Source: CAD feature listing. Evaluate the final solid. Frame: model axes, mm. Give positions to 0.01 mm unless a question says otherwise; leave off trailing zeros. Loops run counter-clockwise (first coordinate to the right, second up) from the corner with the lowest first, then second, coordinate; pieces in that order, holes last. Notation, with made-up numbers: (52.25, 53) - (64.25, 53) arc R32 cw to (64.25, 79) - close; hole circle Ø4 at (1, -21.75). An arc over 180 degrees is marked (long way). Put each result on its own line as item: value.
```python
from build123d import *

# Parameters (mm, degrees)
F0_R     = 7.5
F0_R_2   = 5
F1_DEPTH = 6


with BuildPart() as f1:
    # F0 (on Front) → F1 (new body)
    with BuildSketch(Plane.XZ):
        with BuildLine():
            ThreePointArc((-230, 50), (-244.142136, 44.142136), (-250, 30))
            Line((-250, 30), (-250, -30))
            ThreePointArc((-250, -30), (-244.142136, -44.142136), (-230, -50))
            Line((-230, -50), (230, -50))
            ThreePointArc((230, -50), (244.142136, -44.142136), (250, -30))
            Line((250, -30), (250, 30))
            ThreePointArc((250, 30), (244.142136, 44.142136), (230, 50))
            Line((230, 50), (-230, 50))
        make_face()
        with Locations((-225, 0)):
            Circle(F0_R, mode=Mode.SUBTRACT)
        Circle(F0_R_2, mode=Mode.SUBTRACT)
        with Locations((225, 0)):
            Circle(F0_R, mode=Mode.SUBTRACT)
    extrude(amount=F1_DEPTH)


solid = f1.part
```
1) Section query C-C, the plane y = -3.2. Output: boundary loops of the cut face in (x, z), plus the area to 3 significant figures.
Check result:
outline: (-250, -30) arc R20 ccw to (-230, -50) - (230, -50) arc R20 ccw to (250, -30) - (250, 30) arc R20 ccw to (230, 50) - (-230, 50) arc R20 ccw to (-250, 30) - close; hole circle Ø15 at (-225, 0); hole circle Ø10 at (0, 0); hole circle Ø15 at (225, 0)
area: 49,200 mm²
2) Section query D-D, the plane x = -225. Output: boundary loops of the cut face in (y, z), plus the area to 3 significant figures.
Check result:
outline: (-6, -50) - (0, -50) - (0, -7.5) - (-6, -7.5) - close; (-6, 7.5) - (0, 7.5) - (0, 50) - (-6, 50) - close
area: 510 mm²
3) Pin query (flat end, axial travel): P1, Ø12, axis at x = -193, z = -7, coming from the +Y side; P2, Ø1.5, axis at y = -3, z = 36.5, coming from the +X side. Return the tip coordinate at first contact, or that it passes through.
Check result:
P1: y = 0
P2: x = 249.16
4) Section query A-A, the plane x = 0. Output: boundary loops of the cut face in (y, z).
Check result:
outline: (-6, -50) - (0, -50) - (0, -5) - (-6, -5) - close; (-6, 5) - (0, 5) - (0, 50) - (-6, 50) - close
5) Material intervals for line 1 along Z through (x, y) = (-225, -3.2); line 2 along Z through (x, y) = (0, -2.4); line 3 along X through (y, z) = (-5.6, 31), sorted ascending. Write a range as [from, to].
Check result:
line 1: [-50, -7.5], [7.5, 50]
line 2: [-50, -5], [5, 50]
line 3: [-249.97, 249.97]
6) Mould query, pull axis Z, two halves, no side actions, for faces 1 (the cylindrical face through (217.507, -2.958, 0.33)), 2 (the cylindrical face through (-244.297, -2.958, -43.986)), 3 (the cylindrical face through (-1.08, -2.96, -4.88)), 4 (the cylindrical face through (-243.986, -2.958, 44.297)). Classes: pulls with the +Z half, pulls with the -Z half, needs draft (parallel to the pull), parting line crosses it, or undercut.
Check result:
face 1: undercut
face 2: pulls with the -Z half
face 3: undercut
face 4: pulls with the +Z half
7) Section query B-B, the plane z = 0. Output: boundary loops of the cut face in (x, y), plus the area to 3 significant figures.
Check result:
outline: (-250, -6) - (-232.5, -6) - (-232.5, 0) - (-250, 0) - close; (-217.5, -6) - (-5, -6) - (-5, 0) - (-217.5, 0) - close; (5, -6) - (217.5, -6) - (217.5, 0) - (5, 0) - close; (232.5, -6) - (250, -6) - (250, 0) - (232.5, 0) - close
area: 2,760 mm²
